Here's the drawing with two shaded views (mm, measured from the low corner). I have some questions. Coordinates: 2 decimals unless noted, no trailing zeros. Order: outer loops, then holes, each group sorted by start corner. A loop starts at its lowest first (then second) coordinate and runs counter-clockwise, first axis right, second up. Notation, with made-up numbers: (-37.5, 87.5) - (5.5, 87.5) arc R27 ccw to (5.5, 118.5) - close; hole circle Ø6 at (85, 22). An arc over 180 degrees is marked (long way). Answer as CSV lines item,"result". Start each with the question number.
1. Thinking about a two-plate mould opening in Y: for the marked faces 1, 2, 3 and 4, which applies, released by +Y, released by -Y, zero draft, split by the parting line, or undercut?
2. I want a section at A-A, the plane z = 28. List the corners of the cut face in (x, y) for me (1 decimal).
3. I want a section at C-C, the plane z = 7.5. List the corners of the cut face in (x, y) for me (1 decimal).
4. I need wall thicknesses on probe 1 along Y at (x, z) = (24.5, 20) (1 decimal); probe 2 along Z at (x, y) = (45, 19); probe 3 along X at (y, z) = (25.5, 8). Which ranges of each line are inside material? Lowest first, please.
5. I want a section at B-B, the plane z = 3. List the corners of the cut face in (x, y) for me (1 decimal), and give its area (3 significant figures).
6. For pin 1 (4 mm diameter, centred on x = 5.5, z = 22, fed in from +Y); pin 2 (1 mm diameter, centred on y = 39, z = 23, fed in from +X); pin 3 (1.5 mm diameter, centred on x = 5.5, y = 5.5, fed in from +Z); pin 4 (1 mm diameter, centred on x = 8.5, y = 29, fed in from +Z), each with a flat end and sliding along its axis, tell me the tip position at first contact or that it passes through.
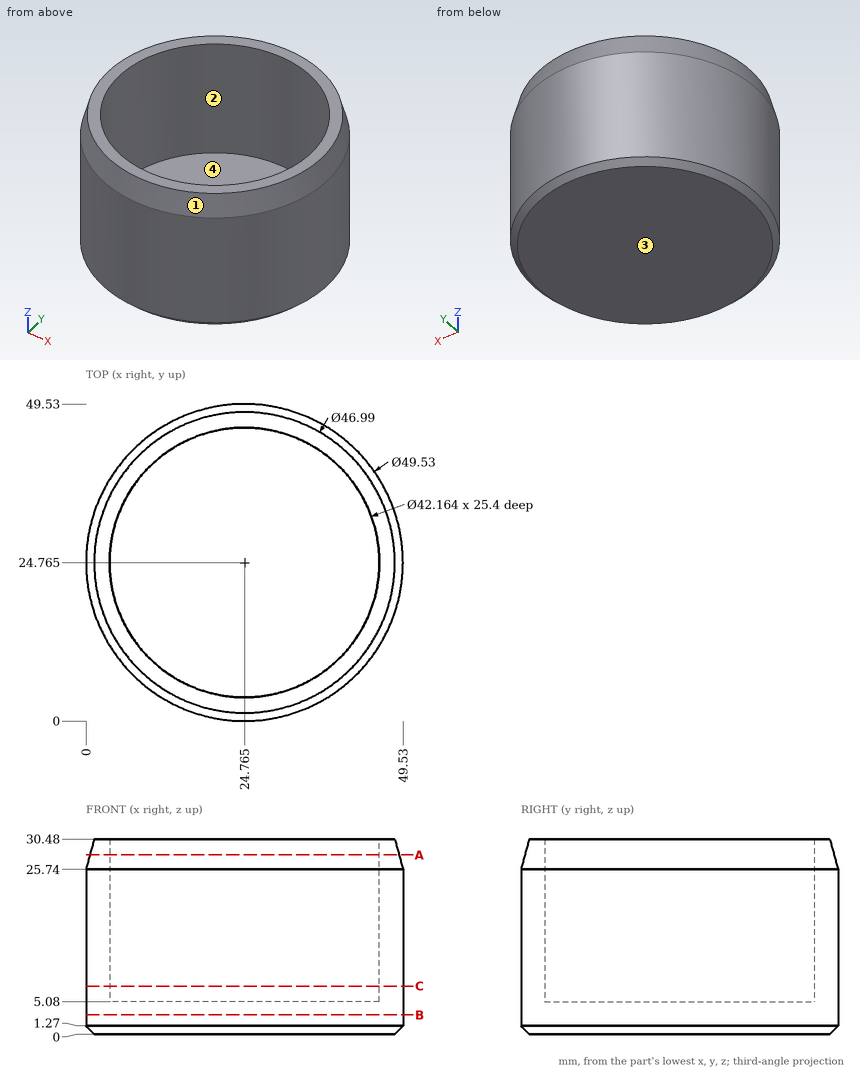
Solved:
1,face 1,"split by the parting line"
1,face 2,"undercut"
1,face 3,"zero draft"
1,face 4,"undercut"
2,outline,"circle Ø48.3 at (24.8, 24.8); hole circle Ø42.2 at (24.8, 24.8)"
3,outline,"circle Ø49.5 at (24.8, 24.8); hole circle Ø42.2 at (24.8, 24.8)"
4,probe 1,"y = 0 to 3.7, 45.8 to 49.5"
4,probe 2,"z = 0 to 5.08"
4,probe 3,"x = 0.01 to 3.7, 45.83 to 49.52"
5,outline,"circle Ø49.5 at (24.8, 24.8)"
5,area,"1,930 mm2"
6,pin 1,"stops at y = 42.52"
6,pin 2,"stops at x = 45.37"
6,pin 3,"passes through"
6,pin 4,"stops at z = 5.08"
